Job drawing, mm, ordinate dimensions from the low corner. One solid piece. Give positions to 0.01 mm unless a question says otherwise; leave off trailing zeros. Order: outer loops, then holes, each group sorted by start corner. A loop starts at its lowest first (then second) coordinate and runs counter-clockwise, first axis right, second up.
Item 1: Wall check: L1, parallel to X at y = 0.6, z = 4 (3 decimals); L2, parallel to Z at x = 24.5, y = 0.9 (3 decimals); L3, parallel to X at y = 0.7, z = 35.5 (3 decimals). Give the ranges that are in metal, low to high.
Item 2: Band-saw the part on A-A on x = 60.5. Give the cut face in (y, z) (3 decimals), plus the area to 4 significant figures.
Item 3: Flat gauge pin, fed straight in: P1, Ø1.8, axis at x = 24.5, z = 5.5, coming from the +Y side. Where does the tip first touch, or does it go through?
Item 4: Band-saw the part on B-B on y = 0.8. Count the separate pieces of the cut face and the enclosed holes in it, plus the area to 3 significant figures.
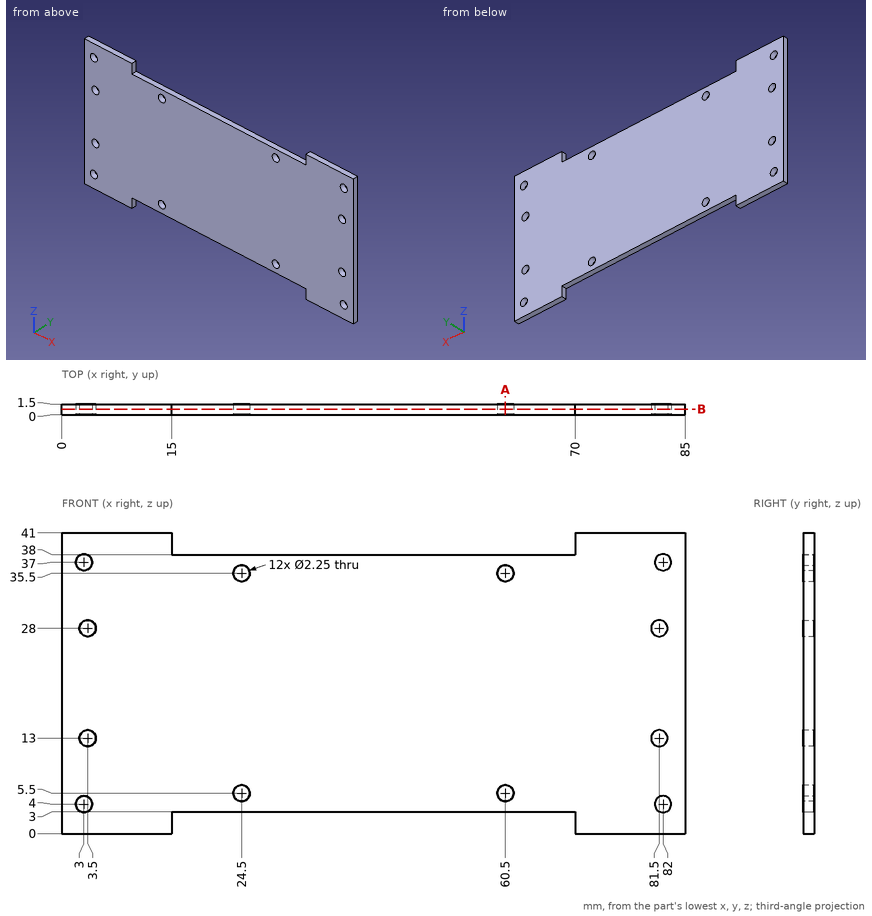
The answers:
1. L1: x = 0 to 1.875, 4.125 to 80.875, 83.125 to 85
1. L2: z = 3 to 4.375, 6.625 to 34.375, 36.625 to 38
1. L3: x = 0 to 23.375, 25.625 to 59.375, 61.625 to 85
2. outline: (0, 3) - (1.5, 3) - (1.5, 4.375) - (0, 4.375) - close; (0, 6.625) - (1.5, 6.625) - (1.5, 34.375) - (0, 34.375) - close; (0, 36.625) - (1.5, 36.625) - (1.5, 38) - (0, 38) - close
2. area: 45.75 mm2
3. P1: passes through
4. separate pieces: 1
4. enclosed holes: 12
4. area: 3,110 mm2
